```python
from build123d import *

# Parameters (mm, degrees)
SKETCH2_RX                    = 25
SKETCH2_RY                    = 15
SKETCH2_RX_2                  = 22.5
SKETCH2_RY_2                  = 12.5
BOSS_EXTRUDE1_DEPTH           = 100
SKETCH8_W                     = 40
SKETCH8_H                     = 40
BOSS_EXTRUDE2_DEPTH           = 20
BOSS_EXTRUDE2_OTHER_WAY_DEPTH = 50
BOSS_EXTRUDE2_OTHER_WAY_TAPER = 5
SKETCH9_W                     = 70
SKETCH9_H                     = 70
BOSS_EXTRUDE3_DEPTH           = 20
SKETCH10_W                    = 60
SKETCH10_H                    = 12
CUT_EXTRUDE1_DEPTH            = 55
CUT_EXTRUDE2_DEPTH            = 155.023239358
CUT_EXTRUDE2_DEPTH_BACK       = 155.023239358
SKETCH11_R                    = 1.75
SKETCH13_R                    = 4
CUT_EXTRUDE3_DEPTH            = 5
CUT_EXTRUDE4_START            = -10
SKETCH14_R                    = 4
CUT_EXTRUDE4_DEPTH            = 10


with BuildPart() as part:
    # Sketch2 → Boss-Extrude1 (new, along a direction that is not the sketch's normal)
    with BuildSketch(Plane(origin=(0, 0, 0), x_dir=(1, 0, 0), z_dir=(0, 1, 0))):
        with Locations(Location((0, 0), (0, 0, -90))):
            Ellipse(SKETCH2_RX, SKETCH2_RY)
        with Locations(Location((0, 0), (0, 0, 90))):
            Ellipse(SKETCH2_RX_2, SKETCH2_RY_2, mode=Mode.SUBTRACT)
    extrude(amount=BOSS_EXTRUDE1_DEPTH, dir=(0, 0.9961946980917453, -0.08715574274766182))

    # Sketch8 → Boss-Extrude2 (add)
    with BuildSketch(Plane(origin=(0, 25, 43.301270189), x_dir=(-1, 0, 0), z_dir=(0, -0.5000000000000041, -0.8660254037844364))):
        with Locations((0, 86.602540378)):
            Rectangle(SKETCH8_W, SKETCH8_H)
    extrude(amount=-BOSS_EXTRUDE2_DEPTH)

    # Sketch8 → Boss-Extrude2 other way (add)
    with BuildSketch(Plane(origin=(0, 25, 43.301270189), x_dir=(-1, 0, 0), z_dir=(0, -0.5000000000000041, -0.8660254037844364))):
        with Locations((0, 86.602540378)):
            Rectangle(SKETCH8_W, SKETCH8_H)
    extrude(amount=BOSS_EXTRUDE2_OTHER_WAY_DEPTH, taper=BOSS_EXTRUDE2_OTHER_WAY_TAPER)

    # Sketch9 → Boss-Extrude3 (add)
    with BuildSketch(Plane(origin=(0, 0, 0), x_dir=(-1, 0, 0), z_dir=(0, -1, 0))):
        Rectangle(SKETCH9_W, SKETCH9_H)
    extrude(amount=BOSS_EXTRUDE3_DEPTH)

    # Sketch10 → Cut-Extrude1 (cut)
    with BuildSketch(Plane.XY.offset(35)):
        with Locations((0, -9.537809852)):
            Rectangle(SKETCH10_W, SKETCH10_H)
    extrude(amount=-CUT_EXTRUDE1_DEPTH, mode=Mode.SUBTRACT)

    # Sketch11 → Cut-Extrude2 (cut, two sides: drawn at the far end of the back side and taken through both)
    with BuildSketch(Plane(origin=(35, 0, 0), x_dir=(0, 0, -1), z_dir=(1, 0, 0)).offset(-CUT_EXTRUDE2_DEPTH_BACK)):
        with Locations((25, -10)):
            Circle(SKETCH11_R)
    extrude(amount=CUT_EXTRUDE2_DEPTH + CUT_EXTRUDE2_DEPTH_BACK, mode=Mode.SUBTRACT)

    # Sketch13 → Cut-Extrude3 (cut)
    with BuildSketch(Plane.ZY.offset(35)):
        with Locations((-25, -10)):
            Circle(SKETCH13_R)
    extrude(amount=-CUT_EXTRUDE3_DEPTH, mode=Mode.SUBTRACT)

    # Sketch14 → Cut-Extrude4 (cut)
    with BuildSketch(Plane(origin=(35, 0, 0), x_dir=(0, 0, -1), z_dir=(1, 0, 0)).offset(CUT_EXTRUDE4_START)):
        with Locations(Location((25, -10, 0), (0, 0, 180))):
            Circle(SKETCH14_R)
    extrude(amount=CUT_EXTRUDE4_DEPTH, mode=Mode.SUBTRACT)


solid = part.part
```
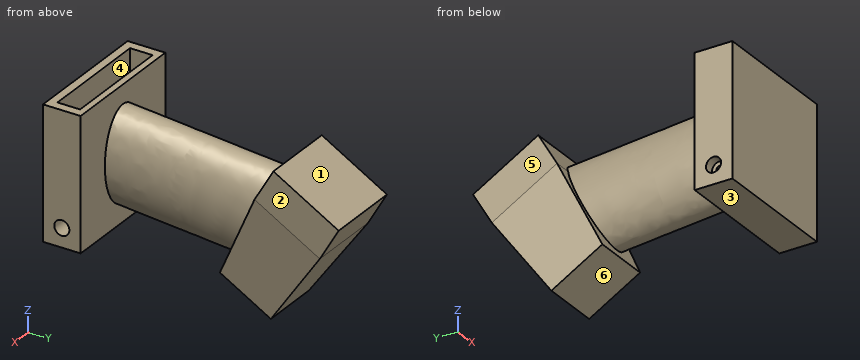
Read the model definition and answer for the solid it produces. Units are mm, in the model's axes. Face numbers are marked on the shaded views. A direction names the side the tool comes from. Round coordinates to 2 decimals unless told otherwise and drop trailing zeros. Write each loop counter-clockwise with the first axis right and the second up, starting at its lowest first coordinate (ties: lowest second). Pieces come first, ordered by that corner, then holes. Notation, with made-up numbers: (-39, 35) -> (3, 35) arc R32 cw to (3, 69) -> close; hole circle Ø5 at (18.5, 72). An arc over 180 degrees is marked (long way). Answer in a Markdown table with one row per item. Add a question column.
1) Determine the mould class of the marked faces 4, 5 and 6 for opening direction X: pulls with the +X half, pulls with the -X half, needs draft (parallel to the pull), parting line crosses it, or undercut.
2) Consider line 1 (X direction, y = -11, z = -2); line 2 (Z direction, x = 32, y = -10); line 3 (Z direction, x = 8, y = -10). Determine where each line is inside the solid, lowest interval first.
3) Find section C-C, the plane z = 19. State how many separate pieces and enclosed holes the cut face has, and give its area (3 significant figures).
4) Which of the six approach directions +Z, -Z, +X, -X, +Y, -Y give full straight-line access (tool end or side, diameter ignored) to the marked faces 1, 2 and 3?
5) Find section A-A, the plane y = -10. Determine the outline of the cut face in (x, z), and give its area (3 significant figures).
6) Given P1, Ø4, axis at y = -8.5, z = -26, coming from the +X side; P2, Ø1.5, axis at y = 58.5, z = -22, coming from the -X side; P3, Ø5, axis at x = -1, z = -7.5, coming from the +Y side, each flat-ended and moving along its own axis, determine where each tip first touches the part or whether it passes through.
7) Find section B-B, the plane x = -24.5. Determine the outline of the cut face in (y, z), and give its area (3 significant figures).
Findings below:
| question | item | result |
|---|---|---|
| 1 | face 4 | undercut |
| 1 | face 5 | pulls with the -X half |
| 1 | face 6 | needs draft |
| 2 | line 1 | -35 to -30, 30 to 35 |
| 2 | line 2 | -35 to -29, -21 to 35 |
| 2 | line 3 | -35 to -26.75, -23.25 to -20 |
| 3 | separate pieces | 2 |
| 3 | enclosed holes | 2 |
| 3 | area | 2,000 mm² |
| 4 | face 1 | +Z, +X, -X, +Y |
| 4 | face 2 | +Z, -Z, +X, +Y |
| 4 | face 3 | -Z, +X, -X, -Y |
| 5 | outline | (-35, -35) -> (35, -35) -> (35, -29) -> (25, -29) -> (25, -26.75) -> (-30, -26.75) -> (-30, -29) -> (-35, -29) -> close; (-35, -21) -> (-30, -21) -> (-30, -23.25) -> (25, -23.25) -> (25, -21) -> (35, -21) -> (35, 35) -> (30, 35) -> (30, -20) -> (-30, -20) -> (-30, 35) -> (-35, 35) -> close |
| 5 | area | 1,290 mm² |
| 6 | P1 | x = 25 |
| 6 | P2 | x = -11.46 |
| 6 | P3 | y = 120.21 |
| 7 | outline | (-20, -35) -> (0, -35) -> (0, 35) -> (-3.54, 35) -> (-3.54, -20) -> (-15.54, -20) -> (-15.54, 35) -> (-20, 35) -> close; hole circle Ø3.5 at (-10, -25) |
| 7 | area | 730 mm² |
